Design review of the part shown in the three views and the two pictorial views. Dimensions are in mm from the part's minimum x, y and z. A direction names the side the tool comes from. Round coordinates to 2 decimals unless told otherwise and drop trailing zeros. Loops run counter-clockwise (first coordinate to the right, second up) from the corner with the lowest first, then second, coordinate; pieces in that order, holes last.
1) Take a section at B-B (z = 0.75). State the section outline as (x, y) points.
2) Insertion check: pin 1 (1.5 mm diameter, centred on y = 21.5, z = 0.5, fed in from -X); pin 2 (0.7 mm diameter, centred on y = 15.5, z = 5, fed in from -X). Each pin has a flat end and moves straight along its axis. Give the tip position at first contact, or say it passes through.
3) Tool access review of the marked faces 1 and 2: name each direction out of +Z, -Z, +X, -X, +Y, -Y from which nothing blocks a thin tool from reaching the whole face with its end or side.
4) Take a section at C-C (x = 10.75). State the section outline as (y, z) points.
5) Take a section at A-A (y = 7.5). State the section outline as (x, z) points, then the cut area to 3 significant figures.
6) Take a section at D-D (y = 47). State the section outline as (x, z) points.
7) Wall thickness on L1, parallel to Y at x = 6, z = 5.2; L2, parallel to X at y = 54, z = 3.1; L3, parallel to Z at x = 3, y = 34: over which ranges is each line inside the solid? List them lowest first.
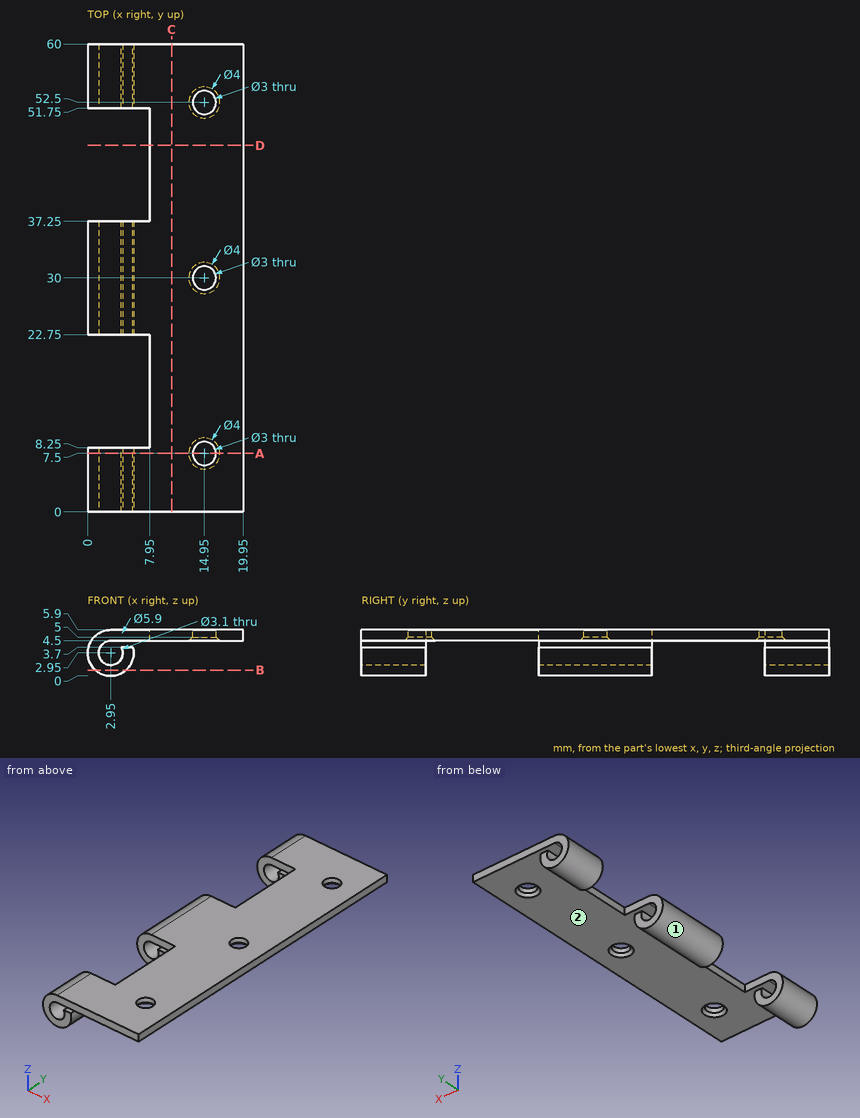
Response:
1. outline: (0.98, 0) - (4.92, 0) - (4.92, 8.25) - (0.98, 8.25) - close; (0.98, 22.75) - (4.92, 22.75) - (4.92, 37.25) - (0.98, 37.25) - close; (0.98, 51.75) - (4.92, 51.75) - (4.92, 60) - (0.98, 60) - close
2. pin 1: passes through
2. pin 2: stops at x = 7.95
3. face 1: +Y, -Y
3. face 2: +X, +Y, -Y
4. outline: (0, 4.5) - (60, 4.5) - (60, 5.9) - (0, 5.9) - close
5. outline: (2.95, 4.5) - (12.95, 4.5) - (13.45, 5) - (13.45, 5.9) - (2.95, 5.9) arc R2.95 ccw (long way) to (5.8, 3.7) - (4.31, 3.7) arc R1.55 cw (long way) to start; (16.45, 5) - (16.95, 4.5) - (19.95, 4.5) - (19.95, 5.9) - (16.45, 5.9) - close
5. area: 35.3 mm2
6. outline: (7.95, 4.5) - (19.95, 4.5) - (19.95, 5.9) - (7.95, 5.9) - close
7. L1: y = 0 to 8.25, 22.75 to 37.25, 51.75 to 60
7. L2: x = 0 to 1.41, 4.49 to 5.9
7. L3: z = 0 to 1.4, 4.5 to 5.9
